Geometry check sheet. Reference: the model listing, model coordinates, mm. Face numbers are marked on the shaded views. A direction names the side the tool comes from. Round coordinates to 2 decimals unless told otherwise and drop trailing zeros. Order: outer loops, then holes, each group sorted by start corner. A loop starts at its lowest first (then second) coordinate and runs counter-clockwise, first axis right, second up.
(1) Sectioned sample at C-C (x = -18.5). Record the boundary of the cut face in (y, z).
(2) Set-up check for the marked faces 1 and 2: record each of +Z, -Z, +X, -X, +Y, -Y from which the full face is reachable in a straight line by a thin tool's end or side.
(3) Sectioned sample at A-A (y = -8). Record the boundary of the cut face in (x, z), plus the area to 3 significant figures.
(4) Material ranges on line 1 along Z through (x, y) = (-44, -12); line 2 along Z through (x, y) = (-37, -18), recorded low to high.
(5) Sectioned sample at D-D (z = 52.5). Record the boundary of the cut face in (x, y), plus the area to 3 significant figures.
(6) Sectioned sample at B-B (z = -40.5). Record the boundary of the cut face in (x, y), plus the area to 3 significant figures.
(7) Release check for a two-part mould opening along Z. For the marked faces 3, 4, 5 and 6 record: +Z half, -Z half, draft (parallel to the pull), parting line (faces both ways), or undercut.
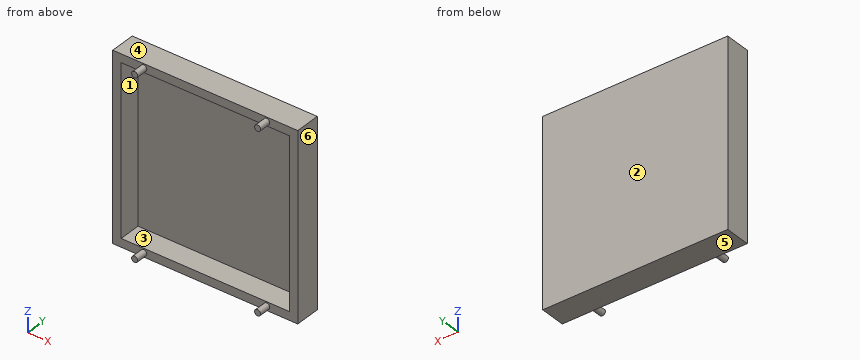
from build123d import *

# Parameters (mm, degrees)
F0_W     = 110
F0_H     = 110
F1_DEPTH = 15
F2_W     = 100
F2_H     = 100
F3_DEPTH = 13
F4_R     = 1.8
F5_DEPTH = 7


with BuildPart() as f1:
    # F0 (on Front) → F1 (new body)
    with BuildSketch(Plane.XZ):
        Rectangle(F0_W, F0_H)
    extrude(amount=F1_DEPTH)

    # F2 (on face) → F3 (cut)
    with BuildSketch(Plane.XZ.offset(15)):
        Rectangle(F2_W, F2_H)
    extrude(amount=-F3_DEPTH, mode=Mode.SUBTRACT)

    # F4 (on face) → F5 (join)
    with BuildSketch(Plane.XZ.offset(15)):
        with Locations((-36.54647, 52.5)):
            Circle(F4_R)
        with Locations((36.54647, 52.5)):
            Circle(F4_R)
        with Locations((-36.54647, -52.5)):
            Circle(F4_R)
        with Locations((36.54647, -52.5)):
            Circle(F4_R)
    extrude(amount=F5_DEPTH)


solid = f1.part
Answer below:
1. outline: (-15, -55) - (0, -55) - (0, 55) - (-15, 55) - (-15, 50) - (-2, 50) - (-2, -50) - (-15, -50) - close
2. face 1: -Y
2. face 2: +Z, -Z, +X, -X, +Y
3. outline: (-55, -55) - (55, -55) - (55, 55) - (-55, 55) - close; hole (-50, -50) - (50, -50) - (50, 50) - (-50, 50) - close
3. area: 2,100 mm2
4. line 1: z = -55 to -50, 50 to 55
4. line 2: z = -54.24 to -50.76, 50.76 to 54.24
5. outline: (-55, -15) - (-38.35, -15) - (-38.35, -22) - (-34.75, -22) - (-34.75, -15) - (34.75, -15) - (34.75, -22) - (38.35, -22) - (38.35, -15) - (55, -15) - (55, 0) - (-55, 0) - close
5. area: 1,700 mm2
6. outline: (-55, -15) - (-50, -15) - (-50, -2) - (50, -2) - (50, -15) - (55, -15) - (55, 0) - (-55, 0) - close
6. area: 350 mm2
7. face 3: undercut
7. face 4: +Z half
7. face 5: -Z half
7. face 6: draft
